from build123d import *

# Parameters (mm, degrees)
BOSS_EXTRU_1_DEPTH      = 133.35
ESQUISSE3_W             = 108.966
ESQUISSE3_H             = 73.152
ENL_V_MAT_EXTRU_1_DEPTH = 222.799600766
ESQUISSE4_R             = 2.286
ENL_V_MAT_EXTRU_2_DEPTH = 172.857608804
CONG_1_R                = 2.54
CONG_2_R                = 2.54
ESQUISSE5_R             = 2.286
ENL_V_MAT_EXTRU_3_DEPTH = 172.857608804
ESQUISSE6_R             = 15.5
ENL_V_MAT_EXTRU_4_DEPTH = 174.176969023
SKETCH1_R               = 17.5
BOSS_EXTRUDE1_DEPTH     = 4
SKETCH2_R               = 13
CUT_EXTRUDE1_DEPTH      = 172.857608804


with BuildPart() as part:
    # Esquisse2 → Boss.-Extru.1 (new body)
    with BuildSketch(Plane.XY):
        Polygon((-64.77, 0), (-80.01, 0), (-80.01, 76.2), (80.01, 76.2), (80.01, 0), (64.77, 0), (64.77, 3.048), (76.962, 3.048), (76.962, 73.152), (-76.962, 73.152), (-76.962, 3.048), (-64.77, 3.048), align=None)
    extrude(amount=BOSS_EXTRU_1_DEPTH)

    # Esquisse3 → Enlèv. mat.-Extru.1 (cut, through all)
    with BuildSketch(Plane.ZY.offset(80.01)):
        with Locations((66.675, 36.576)):
            Rectangle(ESQUISSE3_W, ESQUISSE3_H)
    extrude(amount=-ENL_V_MAT_EXTRU_1_DEPTH, mode=Mode.SUBTRACT)

    # Esquisse4 → Enlèv. mat.-Extru.2 (cut, through all)
    with BuildSketch(Plane(origin=(0, 3.048, 0), x_dir=(1, 0, 0), z_dir=(0, 1, 0))):
        with Locations(Location((73.914, -6.731, 0), (0, 0, 180))):
            Circle(ESQUISSE4_R)
    enl_v_mat_extru_2 = extrude(amount=-ENL_V_MAT_EXTRU_2_DEPTH, mode=Mode.SUBTRACT)

    # Congé1
    cong_1_edges = [part.edges().sort_by_distance(p)[0] for p in [
        (-80.01, 0, 127.254),
        (80.01, 0, 127.254),
        (-80.01, 0, 6.096),
        (80.01, 0, 6.096),
    ]]
    fillet(cong_1_edges, radius=CONG_1_R)

    # Congé2
    cong_2_edges = [part.edges().sort_by_distance(p)[0] for p in [
        (0, 76.2, 0),
        (-80.01, 76.2, 66.675),
        (80.01, 76.2, 66.675),
        (0, 76.2, 133.35),
    ]]
    fillet(cong_2_edges, radius=CONG_2_R)

    # Esquisse5 → Enlèv. mat.-Extru.3 (cut, through all)
    with BuildSketch(Plane(origin=(0, 3.048, 0), x_dir=(1, 0, 0), z_dir=(0, 1, 0))):
        with Locations(Location((73.914, -126.619, 0), (0, 0, 180))):
            Circle(ESQUISSE5_R)
    enl_v_mat_extru_3 = extrude(amount=-ENL_V_MAT_EXTRU_3_DEPTH, mode=Mode.SUBTRACT)

    # Esquisse6 → Enlèv. mat.-Extru.4 (cut, through all)
    with BuildSketch(Plane(origin=(0, 76.2, 0), x_dir=(1, 0, 0), z_dir=(0, 1, 0))):
        with Locations(Location((0, -66.675, 0), (0, 0, 270))):
            Circle(ESQUISSE6_R)
    extrude(amount=-ENL_V_MAT_EXTRU_4_DEPTH, mode=Mode.SUBTRACT)

    # Symétrie1: Enlèv. mat.-Extru.3 across plane
    add(enl_v_mat_extru_3.mirror(Plane(origin=(0, 0, 0), x_dir=(0, 0, 1), z_dir=(1, 0, 0))), mode=Mode.SUBTRACT)

    # Symétrie2: Enlèv. mat.-Extru.2 across plane
    add(enl_v_mat_extru_2.mirror(Plane(origin=(0, 0, 0), x_dir=(0, 0, 1), z_dir=(1, 0, 0))), mode=Mode.SUBTRACT)

    # Sketch1 → Boss-Extrude1 (add)
    with BuildSketch(Plane.XZ.offset(-73.152)):
        with Locations(Location((0, 66.675, 0), (0, 0, 90))):
            Circle(SKETCH1_R)
    extrude(amount=BOSS_EXTRUDE1_DEPTH)

    # Sketch2 → Cut-Extrude1 (cut, through all)
    with BuildSketch(Plane(origin=(0, 73.152, 0), x_dir=(1, 0, 0), z_dir=(0, 1, 0))):
        with Locations(Location((0, -66.675, 0), (0, 0, 270))):
            Circle(SKETCH2_R)
    extrude(amount=-CUT_EXTRUDE1_DEPTH, mode=Mode.SUBTRACT)


solid = part.part
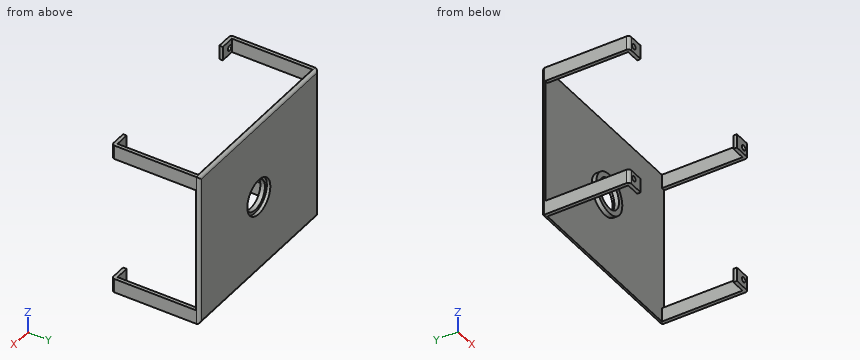
Geometry check sheet. Reference: the model listing, model coordinates, mm. Give positions to 0.01 mm unless a question says otherwise; leave off trailing zeros. Write each loop counter-clockwise with the first axis right and the second up, starting at its lowest first coordinate (ties: lowest second). Pieces come first, ordered by that corner, then holes.
1) Cross-section at D-D (z = 35). Record the boundary of the cut face in (x, y).
Values follow:
outline: (-80.01, 73.15) - (80.01, 73.15) - (80.01, 73.66) arc R2.54 ccw to (77.47, 76.2) - (-77.47, 76.2) arc R2.54 ccw to (-80.01, 73.66) - close
2) Go/stop test with flat-tipped pins: pin 1 Ø3.5 at (x, z) = (-73.914, 126.619) entering from -Y; pin 2 Ø0.9 at (y, z) = (1, 124.5) entering from -X. Record where each tip stops, or that it passes through.
Values follow:
pin 1: stops at y = 73.15
pin 2: stops at x = -79.76
3) Cross-section at A-A (y = 50). Record the boundary of the cut face in (x, z), plus the area to 3 significant figures.
Values follow:
outline: (-80.01, 0) - (-76.96, 0) - (-76.96, 12.19) - (-80.01, 12.19) - close; (-80.01, 121.16) - (-76.96, 121.16) - (-76.96, 133.35) - (-80.01, 133.35) - close; (76.96, 0) - (80.01, 0) - (80.01, 12.19) - (76.96, 12.19) - close; (76.96, 121.16) - (80.01, 121.16) - (80.01, 133.35) - (76.96, 133.35) - close
area: 149 mm2
4) Cross-section at C-C (z = 73.5). Record the boundary of the cut face in (x, y).
Values follow:
outline: (-80.01, 73.15) - (-16.11, 73.15) - (-16.11, 69.15) - (-11.06, 69.15) - (-11.06, 73.15) - (-13.92, 73.15) - (-13.92, 76.2) - (-77.47, 76.2) arc R2.54 ccw to (-80.01, 73.66) - close; (11.06, 69.15) - (16.11, 69.15) - (16.11, 73.15) - (80.01, 73.15) - (80.01, 73.66) arc R2.54 ccw to (77.47, 76.2) - (13.92, 76.2) - (13.92, 73.15) - (11.06, 73.15) - close
5) Cross-section at B-B (x = 0). Record the boundary of the cut face in (y, z) (3 decimals).
Values follow:
outline: (69.152, 49.175) - (73.152, 49.175) - (73.152, 0) - (73.66, 0) arc R2.54 ccw to (76.2, 2.54) - (76.2, 51.175) - (73.152, 51.175) - (73.152, 53.675) - (69.152, 53.675) - close; (69.152, 79.675) - (73.152, 79.675) - (73.152, 82.175) - (76.2, 82.175) - (76.2, 130.81) arc R2.54 ccw to (73.66, 133.35) - (73.152, 133.35) - (73.152, 84.175) - (69.152, 84.175) - close
6) Thickness scan on line 1 (X direction, y = 40, z = 7); line 2 (Y direction, x = -28.5, z = 80); line 3 (Y direction, x = -4, z = 83). Record the ranges inside material, lowest first.
Values follow:
line 1: x = -80.01 to -76.96, 76.96 to 80.01
line 2: y = 73.15 to 76.2
line 3: y = 69.15 to 76.2
